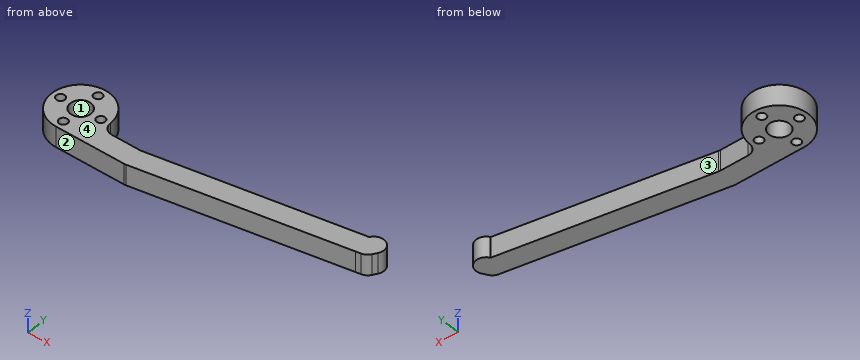
from build123d import *

# Parameters (mm, degrees)
ESQUISSE1_R                  = 8.5
BOSS_EXTRU_1_DEPTH           = 6
BOSS_EXTRU_2_DEPTH           = 6
BOSS_EXTRU_3_DEPTH           = 6
BOSS_EXTRU_4_DEPTH           = 6
ENL_V_MAT_EXTRU_1_DEPTH      = 87.634907569
ENL_V_MAT_EXTRU_1_DEPTH_BACK = 87.634907569
ESQUISSE4_R                  = 3
ESQUISSE4_R_2                = 1.25
CONG_1_R                     = 3


with BuildPart() as part:
    # Esquisse1 → Boss.-Extru.1 (new body)
    with BuildSketch(Plane.XY):
        Circle(ESQUISSE1_R)
    extrude(amount=BOSS_EXTRU_1_DEPTH)

    # Esquisse2 → Boss.-Extru.2 (add)
    with BuildSketch(Plane.XY.offset(6)):
        Polygon((0, -8.5), (20, -8.5), (20, -2.5), (8.124038405, -2.5), align=None)
    extrude(amount=-BOSS_EXTRU_2_DEPTH)

    # Esquisse3 → Boss.-Extru.3 (add)
    with BuildSketch(Plane.XY.offset(6)):
        Polygon((20, -2.5), (79.088465181, 7.91889066), (80.130354247, 2.010044142), (20.524931981, -8.5), (20, -8.5), align=None)
    extrude(amount=-BOSS_EXTRU_3_DEPTH)

    # Esquisse5 → Boss.-Extru.4 (add)
    with BuildSketch(Plane.XY.offset(6)):
        Polygon((80.130354247, 2.010044142), (82.885694629, 2.495884992), (85.784617603, 7.516966871), (80.588465181, 10.516966871), (79.088465181, 7.91889066), align=None)
    extrude(amount=-BOSS_EXTRU_4_DEPTH)

    # Esquisse4 → Enlèv. mat.-Extru.1 (cut, two sides: drawn at the far end of the back side and taken through both)
    with BuildSketch(Plane.XY.offset(6).offset(-ENL_V_MAT_EXTRU_1_DEPTH_BACK)):
        Circle(ESQUISSE4_R)
        with Locations((-6, 0)):
            Circle(ESQUISSE4_R_2)
        with Locations((0, 6)):
            Circle(ESQUISSE4_R_2)
        with Locations((6, 0)):
            Circle(ESQUISSE4_R_2)
        with Locations((0, -6)):
            Circle(ESQUISSE4_R_2)
    extrude(amount=ENL_V_MAT_EXTRU_1_DEPTH + ENL_V_MAT_EXTRU_1_DEPTH_BACK, mode=Mode.SUBTRACT)

    # Congé1
    cong_1_edges = [part.edges().sort_by_distance(p)[0] for p in [
        (20.524931981, -8.5, 3),
        (82.885694629, 2.495884992, 3),
        (85.784617603, 7.516966871, 3),
        (80.588465181, 10.516966871, 3),
        (20, -2.5, 3),
        (8.124038405, -2.5, 3),
    ]]
    fillet(cong_1_edges, radius=CONG_1_R - 0.0001)  # a hair under: the kernel refuses the full size


solid = part.part
CAD build for the part. Positions are in the model's coordinates, mm. Face numbers are marked on the shaded views. A direction names the side the tool comes from. Coordinates: 2 decimals unless noted, no trailing zeros. Write each loop counter-clockwise with the first axis right and the second up, starting at its lowest first coordinate (ties: lowest second). Pieces come first, ordered by that corner, then holes. Notation, with made-up numbers: (49, 34.5) - (88, 34.5) arc R23 cw to (88, 71.5) - close; hole circle Ø11 at (46, 86.25). An arc over 180 degrees is marked (long way). Use a Markdown table: item, result. Add a question column.
Item 1: Drill centre lines: L1, parallel to Y at x = 0, z = 1.5; L2, parallel to Y at x = 19.5, z = 2.5; L3, parallel to Y at x = 10.5, z = 4.45. Where is each one in solid material? Low to high. Write a range as from..to.
Item 2: Band-saw the part on B-B, the plane y = -6. Give the cut face in (x, z), and give its area (3 significant figures).
Item 3: Mould opens along X. For the marked faces 1 and 2 say: pulls with the +X half, pulls with the -X half, needs draft (parallel to the pull), parting line crosses it, or undercut.
Item 4: Band-saw the part on A-A, the plane z = 4.8. Give the number of separate pieces and of enclosed holes in the cut face, and give its area (3 significant figures).
Item 5: Band-saw the part on C-C, the plane x = 6. Give the cut face in (y, z), and give its area (3 significant figures).
Item 6: Band-saw the part on D-D, the plane x = 62.5. Give the cut face in (y, z), and give its area (3 significant figures).
Item 7: 3-axis set-ups, long thin cutter, end or side, ignore diameter. For the marked faces 3 and 4: which of +Z, -Z, +X, -X, +Y, -Y reach the whole face in a straight line?
Item 8: Flat gauge pins, fed straight in: pin 1 (1 mm diameter, centred on y = -4, z = 5, fed in from -X); pin 2 (2 mm diameter, centred on y = 2, z = 3.5, fed in from +X). Where does each tip first touch, or does it go through?
Numbers:
| question | item | result |
|---|---|---|
| 1 | L1 | -8.5..-7.25, -4.75..-3, 3..4.75, 7.25..8.5 |
| 1 | L2 | -8.5..-2.5 |
| 1 | L3 | -8.5..-2.33 |
| 2 | outline | (-6.02, 0) - (-1.25, 0) - (-1.25, 6) - (-6.02, 6) - close; (1.25, 0) - (34.7, 0) - (34.7, 6) - (1.25, 6) - close |
| 2 | area | 229 mm2 |
| 3 | face 1 | undercut |
| 3 | face 2 | needs draft |
| 4 | separate pieces | 1 |
| 4 | enclosed holes | 5 |
| 4 | area | 659 mm2 |
| 5 | outline | (-8.5, 0) - (-1.25, 0) - (-1.25, 6) - (-8.5, 6) - close; (1.25, 0) - (6.02, 0) - (6.02, 6) - (1.25, 6) - close |
| 5 | area | 72.1 mm2 |
| 6 | outline | (-1.1, 0) - (4.99, 0) - (4.99, 6) - (-1.1, 6) - close |
| 6 | area | 36.6 mm2 |
| 7 | face 3 | +Z, -Z, +Y |
| 7 | face 4 | +Z, +X, -X, +Y, -Y |
| 8 | pin 1 | x = -7.75 |
| 8 | pin 2 | x = 83.02 |
